Autodesk Inventor part; units mm, degrees
ref_plane "YZ Plane" through (0, 0, 0) normal (1, 0, 0) x (0, 1, 0)
ref_plane "XZ Plane" through (0, 0, 0) normal (0, 1, 0) x (-1, 0, 0)
ref_plane "XY Plane" through (0, 0, 0) normal (0, 0, 1) x (1, 0, 0)
sketch "Szkic1" plane through (0, 0, 0) normal (0, 1, 0) x (-1, 0, 0)
  circle A0 centre (0, 0) radius 14.1 construction
  line L0 (0, 0) -> (-14.1, 0) construction
  circle A1 centre (0, 0) radius 22.5 construction
  circle A2 centre (-13.2497, 4.8225) radius 1.75
  circle A3 centre (-13.2497, -4.8225) radius 1.75
  circle A4 centre (2.4484, 13.8858) radius 1.75
  circle A5 centre (10.8012, 9.0633) radius 1.75
  circle A6 centre (10.8012, -9.0633) radius 1.75
  circle A7 centre (2.4484, -13.8858) radius 1.75
  circle A8 centre (0, 0) radius 35
  circle A9 centre (-13.2497, 4.8225) radius 3.25
  circle A10 centre (-13.2497, -4.8225) radius 3.25
  circle A11 centre (2.4484, -13.8858) radius 3.25
  circle A12 centre (10.8012, -9.0633) radius 3.25
  circle A13 centre (10.8012, 9.0633) radius 3.25
  circle A14 centre (2.4484, 13.8858) radius 3.25
  line L1 (-9.9997, -4.8225) -> (-9.9997, 4.8225)
  line L2 (-16.4997, 4.8225) -> (-16.4997, -4.8225)
  line L3 (4.0734, -16.7004) -> (12.4262, -11.8779)
  line L4 (9.1762, -6.2487) -> (0.8234, -11.0712)
  line L5 (12.4262, 11.8779) -> (4.0734, 16.7004)
  line L6 (0.8234, 11.0712) -> (9.1762, 6.2487)
  dimension "d0" = 28.2
  dimension "d1" = 3.5
  dimension "d2" = 40
  dimension "d5" = 360
  dimension "d7" = 45
  dimension "d8" = 70
  dimension "d12" = 6.5
  dimension "d15" = 360
  dimension "d29" = 360
sketch "Szkic3" plane through (0, 0, 0) normal (0, 0, 1) x (1, 0, 0)
  arc A0 (0, 35) -> (-35, 0) centre (0, 0) ccw
  line L0 (0, 35) -> (0, 0)
  line L1 (0, 0) -> (-35, 0)
  line L2 (0, -8.4497) -> (0, 50.6985)
  dimension "d19" = 35
revolve "Obrót1" add sketch "Szkic3" angle 360 about axis through (0, -10, 0) along (0, 1, 0)
extrude "Wyciągnięcie proste1" cut sketch "Szkic1" along normal through all contours A2 | A3 | A4 | A5 | A6 | A7 | A9 | L1 A10 L2 A9 | A10 | A11 | A11 L4 A12 L3 | A12 | A13 | A13 L6 A14 L5 | A14
extrude "Wyciągnięcie proste2" add sketch "Szkic1" along normal blind 17.85 contours A9 | L1 A10 L2 A9 | A10 | A11 | A11 L4 A12 L3 | A12 | A13 | A13 L6 A14 L5 | A14
extrude "Wyciągnięcie proste3" cut sketch "Szkic1" along normal blind 7.85 contours A2 | A3 | A4 | A5 | A6 | A7 | A8 | A9 | L1 A10 L2 A9 | A10 | A11 | A11 L4 A12 L3 | A12 | A13 | A13 L6 A14 L5 | A14
properties part number "hemisphere_2"
Design review of the part built by this model. Coordinates are the model's own, in mm. A direction names the side the tool comes from. Round coordinates to 2 decimals unless told otherwise and drop trailing zeros. Write each loop counter-clockwise with the first axis right and the second up, starting at its lowest first coordinate (ties: lowest second). Pieces come first, ordered by that corner, then holes.
Item 1: Draft analysis for pull direction X (two halves, no side actions). For faces 3 (the flat face through (0, 7.85, 0)), 4 (the cylindrical face through (15, 12.78, 4.75)), state which applies: released by +X, released by -X, zero draft, split by the parting line, or undercut.
Item 2: Consider section C-C on y = 19. Give the boundary of the cut face in (x, z).
Item 3: Consider section B-B on z = -10. Give the boundary of the cut face in (x, y), and give its area (3 significant figures).
Item 4: Wall thickness on L1, parallel to Z at x = -10, y = 10.25; L2, parallel to Y at x = -5, z = -14.5; L3, parallel to Z at x = 0, y = 29.25: over which ranges is each line inside the solid? List them lowest first.
Item 5: Consider section D-D on x = -8. Give the boundary of the cut face in (y, z).
Item 6: For pin 1 Ø5.5 at (x, z) = (-6, -9.5) entering from +Y; pin 2 Ø3 at (x, z) = (14, -2) entering from +Y; pin 3 Ø12 at (x, y) = (-4, 12) entering from -Z, all flat-tipped, find the tip position at first contact; note any pin that passes through.
Item 7: For faces 1 (the cylindrical face through (14.998, 12.78, -4.899)), 2 (the cylindrical face through (13.32, 25.41, 8.07)), list the 3-axis set-ups (+Z, -Z, +X, -X, +Y, -Y) from which the entire face can be reached by the end or side of a thin tool; tool diameter is ignored.
Item 8: Consider section A-A on y = 12.5. Give the boundary of the cut face in (x, z).
Check values:
1. face 3: zero draft
1. face 4: undercut
2. outline: circle Ø58.79 at (0, 0); hole (-12.43, -11.88) - (-4.07, -16.7) arc R3.25 ccw to (-0.82, -11.07) - (-9.18, -6.25) arc R3.25 ccw to start; hole (-12.43, 11.88) arc R3.25 ccw to (-9.18, 6.25) - (-0.82, 11.07) arc R3.25 ccw to (-4.07, 16.7) - close; hole (10, -4.82) arc R3.25 ccw to (16.5, -4.82) - (16.5, 4.82) arc R3.25 ccw to (10, 4.82) - close
3. outline: (-32.61, 7.85) - (-12.28, 7.85) - (-12.28, 17.85) - (-13.91, 17.85) - (-13.91, 30.52) arc R33.54 ccw to start; (-9.32, 7.85) - (32.61, 7.85) arc R33.54 ccw to (-2.68, 33.43) - (-2.68, 17.85) - (-9.32, 17.85) - close
3. area: 1,050 mm2
4. L1: z = -31.94 to -10.62, -7.51 to 7.51, 10.62 to 31.94
4. L2: y = 7.85 to 17.85
4. L3: z = -19.22 to -16.02, -11.75 to 11.75, 16.02 to 19.22
5. outline: (7.85, -33.16) arc R34.07 ccw to (30.87, -14.43) - (17.85, -14.43) - (17.85, -6.93) - (33.36, -6.93) arc R34.07 ccw to (33.36, 6.93) - (17.85, 6.93) - (17.85, 14.43) - (30.87, 14.43) arc R34.07 ccw to (7.85, 33.16) - close
6. pin 1: stops at y = 33.96
6. pin 2: stops at y = 17.85
6. pin 3: stops at z = -34.11
7. face 1: +Y, -Y
7. face 2: +Y
8. outline: circle Ø65.38 at (0, 0); hole circle Ø3.5 at (-10.8, -9.06); hole circle Ø3.5 at (-10.8, 9.06); hole circle Ø3.5 at (-2.45, -13.89); hole circle Ø3.5 at (-2.45, 13.89); hole circle Ø3.5 at (13.25, -4.82); hole circle Ø3.5 at (13.25, 4.82)
